```python
from build123d import *

# Parameters (mm, degrees)
ESTRUSIONE_ESTRUSIONE1_DEPTH       = 75
SCHIZZO2_R                         = 53
TAGLIO_ESTRUSIONE1_DEPTH           = 75
SCHIZZO3_R                         = 60
TAGLIO_ESTRUSIONE2_DEPTH           = 28
FORO_PER_VITE_M3_1_D               = 5.6
FORO_PER_VITE_M3_1_DEPTH           = 8.1
FORO_PER_VITE_M3_1_TIP             = 1.682409733
FORO_PER_VITE_M3_1_ON_FACE_2_D     = 5.6
FORO_PER_VITE_M3_1_ON_FACE_2_DEPTH = 8.1
FORO_PER_VITE_M3_1_ON_FACE_2_TIP   = 1.682409733


with BuildPart() as part:
    # Schizzo1 → Estrusione-Estrusione1 (new body)
    with BuildSketch(Plane.XY):
        Polygon((-6, 38.5), (38.5, 38.5), (38.5, 44), (-11.5, 44), (-68.8406431, 3.849649455), (-65.972760918, -0.246110766), (-26.428417773, 27.443136398), (-16.428417773, 27.443136398), (-6, 17.014718626), (-6, 5), (-1, 0), (0, 0), (20.5, 0), (20.5, 25.5), (0, 25.5), (-6, 25.5), (-8.5, 28), (-8.5, 36), align=None)
    extrude(amount=ESTRUSIONE_ESTRUSIONE1_DEPTH)

    # Schizzo2 → Taglio-Estrusione1 (cut)
    with BuildSketch(Plane(origin=(0, 44, 0), x_dir=(1, 0, 0), z_dir=(0, 1, 0))):
        with Locations((61.1, -37.5)):
            Circle(SCHIZZO2_R)
    extrude(amount=-TAGLIO_ESTRUSIONE1_DEPTH, mode=Mode.SUBTRACT)

    # Schizzo3 → Taglio-Estrusione2 (cut)
    with BuildSketch(Plane.XZ):
        with Locations((61.1, 37.5)):
            Circle(SCHIZZO3_R)
    extrude(amount=-TAGLIO_ESTRUSIONE2_DEPTH, mode=Mode.SUBTRACT)

    # Foro per Vite M3-1
    with Locations(Plane(origin=(4.718442753, 5, 16.9787914), x_dir=(-0.342020143326, 0, 0.939692620786), z_dir=(0.939692620786, 0, 0.342020143326))):
        with Locations((0, 0)):
            Hole(FORO_PER_VITE_M3_1_D / 2, depth=FORO_PER_VITE_M3_1_DEPTH)
            with Locations((0, 0, -(FORO_PER_VITE_M3_1_DEPTH + FORO_PER_VITE_M3_1_TIP / 2))):  # 118° drill point
                Cone(0, FORO_PER_VITE_M3_1_D / 2, FORO_PER_VITE_M3_1_TIP, mode=Mode.SUBTRACT)

    # Foro per Vite M3-1 on face 2
    with Locations(Plane(origin=(4.718442753, 5, 58.0212086), x_dir=(0.342019894889, 0, 0.939692711209), z_dir=(0.939692711209, 0, -0.342019894889))):
        with Locations((0, 0)):
            Hole(FORO_PER_VITE_M3_1_ON_FACE_2_D / 2, depth=FORO_PER_VITE_M3_1_ON_FACE_2_DEPTH)
            with Locations((0, 0, -(FORO_PER_VITE_M3_1_ON_FACE_2_DEPTH + FORO_PER_VITE_M3_1_ON_FACE_2_TIP / 2))):  # 118° drill point
                Cone(0, FORO_PER_VITE_M3_1_ON_FACE_2_D / 2, FORO_PER_VITE_M3_1_ON_FACE_2_TIP, mode=Mode.SUBTRACT)


solid = part.part
```
Can you work these out from the model? Positions are in its coordinate system, mm. A direction names the side the tool comes from. Give positions to 0.01 mm unless a question says otherwise; leave off trailing zeros. Order: outer loops, then holes, each group sorted by start corner. A loop starts at its lowest first (then second) coordinate and runs counter-clockwise, first axis right, second up. Notation, with made-up numbers: M 69,77.25 L 73,77.25 A15 cw 73,88.25 Z; hole C -2,63.25 d5. An arc over 180 degrees is marked long. One line per item, written item: value.
1) On a 3-axis mill with a long thin cutter (end or side, diameter ignored), from which of +Z, -Z, +X, -X, +Y, -Y can I reach the whole of each face in a straight line? I mean faces 4 (the face through (0, 0, 37)), 5 (the face through (-67.427, 1.83, 36.975)), 6 (the face through (0, 25.5, 37)), 7 (the face through (1.103, 12.572, 38.067)), 8 (the face through (-11.287, 22.302, 36.975)). Say none if no direction works.
Answer sheet:
face 4: +Z, -Z, +X, -Y
face 5: +Z, -Z, -X, -Y
face 6: +Z, -Z, +X
face 7: +X, -Y
face 8: +Z, -Z, -Y
2) Please list where these lines run through material, in increasing order: line 1 along Y through (x, z) = (3, 64); line 2 along Y through (x, z) = (-3, 38); line 3 along X through (y, z) = (6, 66).
Answer sheet:
line 1: y = 0 to 25.5, 38.5 to 44
line 2: y = 2 to 25.5, 38.5 to 44
line 3: x = -65.77 to -57.05, -6 to 8.3
3) I want a section at A-A, the plane y = 11. List the corners of the cut face in (x, z) for me.
Answer sheet:
outline: M -58.63,0 L -49.91,0 L -49.91,75 L -58.63,75 Z; M -6,0 L 14.26,0 A60 cw 14.26,75 L -6,75 Z
4) I want a section at C-C, the plane y = 30.5. List the corners of the cut face in (x, z) for me.
Answer sheet:
outline: M -30.78,0 L -8.5,0 L -8.5,75 L -30.78,75 Z
5) I want a section at B-B, the plane z = 30.5. List the corners of the cut face in (x, y) for me.
Answer sheet:
outline: M -68.84,3.85 L -65.97,-0.25 L -26.43,27.44 L -16.43,27.44 L -6,17.01 L -6,5 L -1,0 L 1.51,0 L 1.51,25.5 L -6,25.5 L -8.5,28 L -8.5,36 L -6,38.5 L 8.56,38.5 L 8.56,44 L -11.5,44 Z
6) I want a section at D-D, the plane x = -35. List the corners of the cut face in (y, z) for me, plus the area to 3 significant figures.
Answer sheet:
outline: M 21.44,0 L 27.55,0 L 27.55,75 L 21.44,75 Z
area: 458 mm^2
7) For P1, Ø15, axis at x = 10, z = 31, coming from the -Y side; P2, Ø6, axis at x = -22.5, y = 39, coming from the -Z side; P3, Ø3, axis at x = -48, z = 56.5, coming from the -Y side; P4, Ø12, axis at y = 33.5, z = 32.5, coming from the -X side, each with a flat end and sliding along its axis, tell me the tip position at first contact or that it passes through.
Answer sheet:
P1: stops at y = 38.5
P2: stops at z = 0
P3: stops at y = 11.29
P4: stops at x = -35.06
8) We'd pull the mould along Z, two halves only. Please class faces 1 (the face through (-9.11, 20.34, 0)), 2 (the face through (-39.769, 24.206, 36.975)), 3 (the face through (-4.29, 4.59, 13.98)): released by +Z, released by -Z, zero draft, split by the parting line, or undercut.
Answer sheet:
face 1: released by -Z
face 2: zero draft
face 3: undercut
